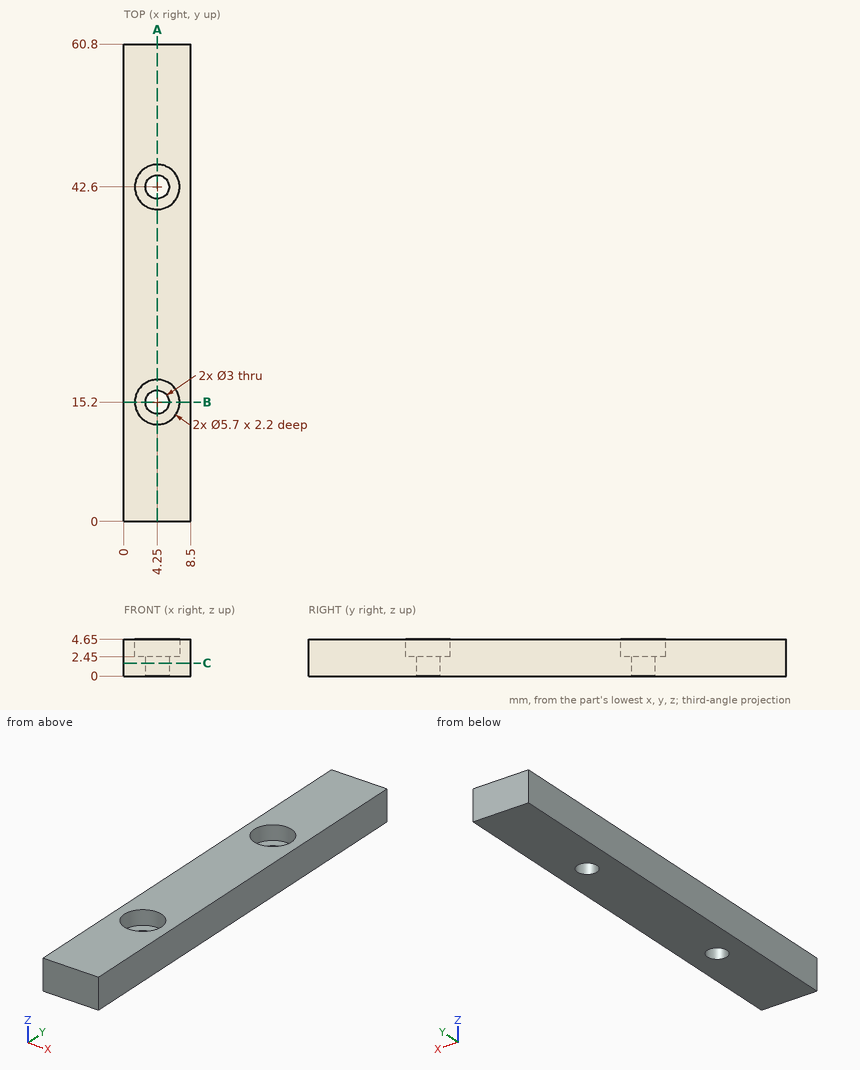
Geometry check sheet. Reference: drawing and pictorial views, mm from the part's lowest x, y, z. Give positions to 0.01 mm unless a question says otherwise; leave off trailing zeros. Write each loop counter-clockwise with the first axis right and the second up, starting at its lowest first coordinate (ties: lowest second). Pieces come first, ordered by that corner, then holes.
Item 1: Cross-section at A-A (x = 4.25). Enter the section's corners in (y, z), and give its area (3 significant figures).
Item 2: Scan lines: L1, parallel to Y at x = 4.25, z = 0.6; L2, parallel to Y at x = 3, z = 0.9; L3, parallel to X at y = 42.6, z = 1.25. Record each from-to range of solid material in increasing order.
Item 3: Cross-section at C-C (z = 1.65). Enter the section's corners in (x, y), and give its area (3 significant figures).
Item 4: Cross-section at B-B (y = 15.2). Enter the section's corners in (x, z), and give its area (3 significant figures).
Item 5: Gauge pin test, flat end, axial feed: pin 1 (2.5 mm diameter, centred on x = 4.25, y = 15.2, fed in from +Z). Record the tip position at first contact, or that the pin passes through.
Report:
1. outline: (0, 0) - (13.7, 0) - (13.7, 2.45) - (12.35, 2.45) - (12.35, 4.65) - (0, 4.65) - close; (16.7, 0) - (41.1, 0) - (41.1, 2.45) - (39.75, 2.45) - (39.75, 4.65) - (18.05, 4.65) - (18.05, 2.45) - (16.7, 2.45) - close; (44.1, 0) - (60.8, 0) - (60.8, 4.65) - (45.45, 4.65) - (45.45, 2.45) - (44.1, 2.45) - close
1. area: 243 mm2
2. L1: y = 0 to 13.7, 16.7 to 41.1, 44.1 to 60.8
2. L2: y = 0 to 14.37, 16.03 to 41.77, 43.43 to 60.8
2. L3: x = 0 to 2.75, 5.75 to 8.5
3. outline: (0, 0) - (8.5, 0) - (8.5, 60.8) - (0, 60.8) - close; hole circle Ø3 at (4.25, 15.2); hole circle Ø3 at (4.25, 42.6)
3. area: 503 mm2
4. outline: (0, 0) - (2.75, 0) - (2.75, 2.45) - (1.4, 2.45) - (1.4, 4.65) - (0, 4.65) - close; (5.75, 0) - (8.5, 0) - (8.5, 4.65) - (7.1, 4.65) - (7.1, 2.45) - (5.75, 2.45) - close
4. area: 19.6 mm2
5. pin 1: passes through
